Autodesk Inventor part; units mm, degrees
ref_plane "YZ Plane" through (0, 0, 0) normal (1, 0, 0) x (0, 1, 0)
ref_plane "XZ Plane" through (0, 0, 0) normal (0, 1, 0) x (-1, 0, 0)
ref_plane "XY Plane" through (0, 0, 0) normal (0, 0, 1) x (1, 0, 0)
sketch "Skizze1" plane through (0, 0, 0) normal (0, 0, 1) x (1, 0, 0)
  line L0 (-27, -12) -> (27, -12)
  line L1 (27, -12) -> (27, 12)
  line L2 (27, 12) -> (-27, 12)
  line L3 (-27, 12) -> (-27, -12)
  circle A0 centre (-20, 0) radius 3.05
  circle A1 centre (20, 0) radius 3.05
  point P0 (0, 0)
  dimension "d0" = 54
  dimension "d1" = 24
  dimension "d2" = 12
  dimension "d3" = 27
  dimension "d4" = 6.1
  dimension "d5" = 20
  dimension "d6" = 12
  dimension "d7" = 20
  dimension "d8" = 6.1
  dimension "d9" = 12
extrude "Extrusion1" add sketch "Skizze1" along normal blind 4
sketch "Skizze2" plane through (0, 0, 4) normal (0, 0, 1) x (1, 0, 0)
  circle A0 centre (-20, 0) radius 3.05
  circle A1 centre (20, 0) radius 3.05
  circle A2 centre (-20, 0) radius 7
  circle A3 centre (-20, 0) radius 3.05
  circle A4 centre (20, 0) radius 3.05
  circle A5 centre (20, 0) radius 7
  point P0 (0, 0)
  dimension "d3" = 27
  dimension "d12" = 6.1
  dimension "d13" = 14
  dimension "d14" = 6.1
  dimension "d15" = 14
extrude "Extrusion2" add sketch "Skizze2" along normal blind 5
properties part number "B Oben"
The model under review builds one solid part; all positions refer to its coordinate system, in mm. A direction names the side the tool comes from. Give positions to 0.01 mm unless a question says otherwise; leave off trailing zeros. Write each loop counter-clockwise with the first axis right and the second up, starting at its lowest first coordinate (ties: lowest second). Pieces come first, ordered by that corner, then holes. Notation, with made-up numbers: (49.5, 7) - (96.5, 7) arc R31 ccw to (96.5, 46) - close; hole circle Ø5 at (59.5, 48.5). An arc over 180 degrees is marked (long way). Answer in a Markdown table with one row per item. Add a question column.
1. Tool access review of faces 1 (the cylindrical face through (13, 0, 6)), 2 (the cylindrical face through (22.817, 1.168, 4.437)): name each direction out of +Z, -Z, +X, -X, +Y, -Y from which nothing blocks a thin tool from reaching the whole face with its end or side.
2. We need section A-A on x = -20. Write out the cut boundary in (y, z), then the cut area to 3 significant figures.
3. We need section B-B on z = 4.5. Write out the cut boundary in (x, y).
4. We need section D-D on y = 6.25. Write out the cut boundary in (x, z).
5. Insertion check: P1, Ø1.5, axis at x = 8, y = -1, coming from the +Z side. The pin has a flat end and moves straight along its axis. Give the tip position at first contact, or say it passes through.
6. We need section C-C on y = -0.75. Write out the cut boundary in (x, z).
7. Draft analysis for pull direction X (two halves, no side actions). For faces 3 (the flat face through (27, 0, 2)), 4 (the cylindrical face through (-27, 0, 6)), 5 (the flat face through (23, -1.5, 9)), state which applies: +X half, -X half, draft (parallel to the pull), parting line (faces both ways), or undercut.
8. Wall thickness on line 1 along Y through (x, z) = (20, 6.75); line 2 along X through (y, z) = (-0.5, 6.5); line 3 along Z through (x, y) = (13.5, -6.5): over which ranges is each line inside the solid? List them lowest first. Write a range as [from, to].
Ans:
| question | item | result |
|---|---|---|
| 1 | face 1 | +Z |
| 1 | face 2 | +Z, -Z |
| 2 | outline | (-12, 0) - (-3.05, 0) - (-3.05, 9) - (-7, 9) - (-7, 4) - (-12, 4) - close; (3.05, 0) - (12, 0) - (12, 4) - (7, 4) - (7, 9) - (3.05, 9) - close |
| 2 | area | 111 mm^2 |
| 3 | outline | circle Ø14 at (-20, 0); circle Ø14 at (20, 0); hole circle Ø6.1 at (-20, 0); hole circle Ø6.1 at (20, 0) |
| 4 | outline | (-27, 0) - (27, 0) - (27, 4) - (23.15, 4) - (23.15, 9) - (16.85, 9) - (16.85, 4) - (-16.85, 4) - (-16.85, 9) - (-23.15, 9) - (-23.15, 4) - (-27, 4) - close |
| 5 | P1 | stops at z = 4 |
| 6 | outline | (-27, 0) - (-22.96, 0) - (-22.96, 9) - (-26.96, 9) - (-26.96, 4) - (-27, 4) - close; (-17.04, 0) - (17.04, 0) - (17.04, 9) - (13.04, 9) - (13.04, 4) - (-13.04, 4) - (-13.04, 9) - (-17.04, 9) - close; (22.96, 0) - (27, 0) - (27, 4) - (26.96, 4) - (26.96, 9) - (22.96, 9) - close |
| 7 | face 3 | +X half |
| 7 | face 4 | undercut |
| 7 | face 5 | draft |
| 8 | line 1 | y = [-7, -3.05], [3.05, 7] |
| 8 | line 2 | x = [-26.98, -23.01], [-16.99, -13.02], [13.02, 16.99], [23.01, 26.98] |
| 8 | line 3 | z = [0, 4] |
